Source: CAD feature listing. Evaluate the final solid. Frame: model axes, mm. Face numbers are marked on the shaded views. A direction names the side the tool comes from. Give positions to 0.01 mm unless a question says otherwise; leave off trailing zeros. Loops run counter-clockwise (first coordinate to the right, second up) from the corner with the lowest first, then second, coordinate; pieces in that order, holes last. Notation, with made-up numbers: M 25.25,-8.75 L 43.25,-8.75 A21 ccw 43.25,8.25 Z; hole C 35.5,-8.75 d5. An arc over 180 degrees is marked long. Put each result on its own line as item: value.
Autodesk Inventor part; units mm, degrees
ref_plane "YZ Plane" through (0, 0, 0) normal (1, 0, 0) x (0, 1, 0)
ref_plane "XZ Plane" through (0, 0, 0) normal (0, 1, 0) x (-1, 0, 0)
ref_plane "XY Plane" through (0, 0, 0) normal (0, 0, 1) x (1, 0, 0)
sketch "Sketch1" plane through (0, 0, 0) normal (0, 0, 1) x (1, 0, 0)
  circle A0 centre (0, 0) radius 101.6
  circle A1 centre (0, 0) radius 127
  dimension "d0" = 203.2
  dimension "d1" = 25.4
extrude "Extrusion1" add sketch "Sketch1" along normal mid plane 101.6
sketch "Sketch2" plane through (0, 0, 50.8) normal (0, 0, 1) x (1, 0, 0)
  circle A0 centre (0, 0) radius 127
  line L0 (-14.3768, 126.1836) -> (-6.8242, 107.95)
  line L1 (-6.8242, 107.95) -> (6.8242, 107.95)
  line L2 (6.8242, 107.95) -> (14.3768, 126.1836)
  line L3 (0, 107.95) -> (0, 128.4311) construction
  line L4 (-14.3768, 126.1836) -> (0, 0) construction
  line L5 (0, 0) -> (14.3768, 126.1836) construction
  arc A1 (14.3768, 126.1836) -> (-14.3768, 126.1836) centre (0, 0) ccw
  dimension "d4" = 19.05
  dimension "d5" = 45
  dimension "d6" = 13
extrude "Extrusion2" cut sketch "Sketch2" against normal through all contours L2 L1 L0 A0 picked at (1.6005, 114.2697)
pattern_circular "Circular Pattern1" count 24 over 360 about axis through (0, 0, 0) along (0, 0, 1) of "Extrusion2"
properties part number "NASA-20-HUB-TRD-01" material "PET Plastic"
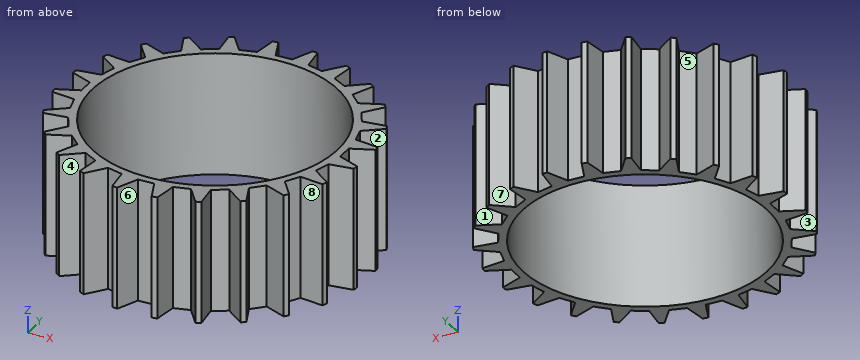
1. Contact query for flat-ended pins moving along their axis: P1, Ø3, axis at y = 25.5, z = -9.5, coming from the +X side; P2, Ø1.5, axis at x = -93.5, z = 37.5, coming from the -Y side; P3, Ø3, axis at x = -19.5, z = -16, coming from the +Y side. Output: stop coordinate, or through.
Found:
P1: x = 105.33
P2: y = -76.93
P3: y = 125.72
2. Draft query along Y for the marked faces 6, 7 and 8. Return one class per face: pulls with the +Y half, pulls with the -Y half, needs draft (parallel to the pull), parting line crosses it, or undercut.
Found:
face 6: pulls with the -Y half
face 7: pulls with the +Y half
face 8: undercut
3. Section query A-A (y = 0). Output: boundary loops of the cut face in (x, z).
Found:
outline: M -107.95,-50.8 L -101.6,-50.8 L -101.6,50.8 L -107.95,50.8 Z; M 101.6,-50.8 L 107.95,-50.8 L 107.95,50.8 L 101.6,50.8 Z
4. Material intervals for line 1 (Y direction, x = 0, z = -4); line 2 (Y direction, x = -13.5, z = 38); line 3 (Y direction, x = -78, z = 1.5), sorted ascending. Write a range as from..to.
Found:
line 1: -107.95..-101.6, 101.6..107.95
line 2: -124.07..-100.7, 100.7..124.07
line 3: -100.22..-96.83, -74.66..-65.1, 65.1..74.66, 96.83..100.22
5. Access query for the marked faces 1, 2, 3, 4 and 5. Directions: +Z, -Z, +X, -X, +Y, -Y. A direction counts if a zero-diameter tool reaches every point of the face in a straight line with its end or side. Return the directions, or none.
Found:
face 1: +Z, -Z, +Y
face 2: +Z, -Z, +X
face 3: +Z, -Z, -X
face 4: +Z, -Z, -Y
face 5: +Z, -Z
6. Section query C-C (y = 111.5). Output: boundary loops of the cut face in (x, z), plus the area to 3 significant figures.
Found:
outline: M -49.99,-50.8 L -41.43,-50.8 L -41.43,50.8 L -49.99,50.8 Z; M -20.63,-50.8 L -8.29,-50.8 L -8.29,50.8 L -20.63,50.8 Z; M 8.29,-50.8 L 20.63,-50.8 L 20.63,50.8 L 8.29,50.8 Z; M 41.43,-50.8 L 49.99,-50.8 L 49.99,50.8 L 41.43,50.8 Z
area: 4,240 mm^2
